Model file for the job. Use its own axes, mm. A direction names the side the tool comes from. Coordinates: 2 decimals unless noted, no trailing zeros. Loops run counter-clockwise (first coordinate to the right, second up) from the corner with the lowest first, then second, coordinate; pieces in that order, holes last. Notation, with made-up numbers: (49.25, -24.5) -> (60.25, -24.5) arc R32 cw to (60.25, 3.5) -> close; hole circle Ø5 at (40.5, -39). An arc over 180 degrees is marked (long way). Use one line per item in the form item = value.
```python
from build123d import *

# Parameters (mm, degrees)
BOSS_EXTRUDE1_DEPTH = 19.05


with BuildPart() as part:
    # Sketch1 → Boss-Extrude1 (new body)
    with BuildSketch(Plane.XY):
        with BuildLine():
            Line((0, 101.6), (0, 0))
            Line((0, 0), (508, 0))
            Line((508, 0), (508, 101.6))
            Line((508, 101.6), (444.5, 101.6))
            Line((444.5, 101.6), (444.5, 88.540005908))
            ThreePointArc((444.5, 88.540005908), (431.8, 75.840005908), (419.1, 88.540005908))
            Line((419.1, 88.540005908), (419.1, 101.6))
            Line((419.1, 101.6), (88.9, 101.6))
            Line((88.9, 101.6), (88.9, 88.9))
            ThreePointArc((88.9, 88.9), (76.2, 76.2), (63.5, 88.9))
            Line((63.5, 88.9), (63.5, 101.6))
            Line((63.5, 101.6), (0, 101.6))
        make_face()
    extrude(amount=BOSS_EXTRUDE1_DEPTH)


solid = part.part
```
Q1. Band-saw the part on B-B, the plane z = 8.5. Write the cut outline in (x, y).
Result:
outline = (0, 0) -> (508, 0) -> (508, 101.6) -> (444.5, 101.6) -> (444.5, 88.54) arc R12.7 cw to (419.1, 88.54) -> (419.1, 101.6) -> (88.9, 101.6) -> (88.9, 88.9) arc R12.7 cw to (63.5, 88.9) -> (63.5, 101.6) -> (0, 101.6) -> close
Q2. Band-saw the part on D-D, the plane x = 431.8. Write the cut outline in (y, z).
Result:
outline = (0, 0) -> (75.84, 0) -> (75.84, 19.05) -> (0, 19.05) -> close
Q3. Mould opens along X. For faces 1 (the face through (444.5, 95, 9)), 2 (the face through (256, 101.6, 9)), 3 (the face through (432.079, 75.843, 9.392)), 4 (the face through (0, 52, 9)) say: released by +X, released by -X, zero draft, split by the parting line, or undercut.
Result:
face_1 = undercut
face_2 = zero draft
face_3 = undercut
face_4 = released by -X
Q4. Pin check, flat tip, straight feed: pin 1 Ø3 at (x, z) = (77.5, 10) entering from +Y. Stop position of the tip, or through.
Result:
pin_1 = 76.51
Q5. Wall check: line 1 along X through (y, z) = (87.5, 1.25); line 2 along X through (y, z) = (88, 1.25); line 3 along Y through (x, z) = (78, 11.5). Give the ranges that are in metal, low to high.
Result:
line_1 = 0 to 63.58, 88.82 to 419.14, 444.46 to 508
line_2 = 0 to 63.53, 88.87 to 419.11, 444.49 to 508
line_3 = 0 to 76.33
Q6. Which spindle directions (+Z, -Z, +X, -X, +Y, -Y) get a long thin tool onto all of the face, cutting with end or side? Do faces 5 (the face through (63.5, 95, 9)), 6 (the face through (477, 101.6, 9)). Say none if no direction does.
Result:
face_5 = +Z, -Z, +Y
face_6 = +Z, -Z, +X, -X, +Y
Q7. Band-saw the part on C-C, the plane x = 76.2. Write the cut outline in (y, z), and give its area (3 significant figures).
Result:
outline = (0, 0) -> (76.2, 0) -> (76.2, 19.05) -> (0, 19.05) -> close
area = 1,450 mm2
Q8. Band-saw the part on A-A, the plane y = 84. Write the cut outline in (x, z).
Result:
outline = (0, 0) -> (64.48, 0) -> (64.48, 19.05) -> (0, 19.05) -> close; (87.92, 0) -> (419.94, 0) -> (419.94, 19.05) -> (87.92, 19.05) -> close; (443.66, 0) -> (508, 0) -> (508, 19.05) -> (443.66, 19.05) -> close
